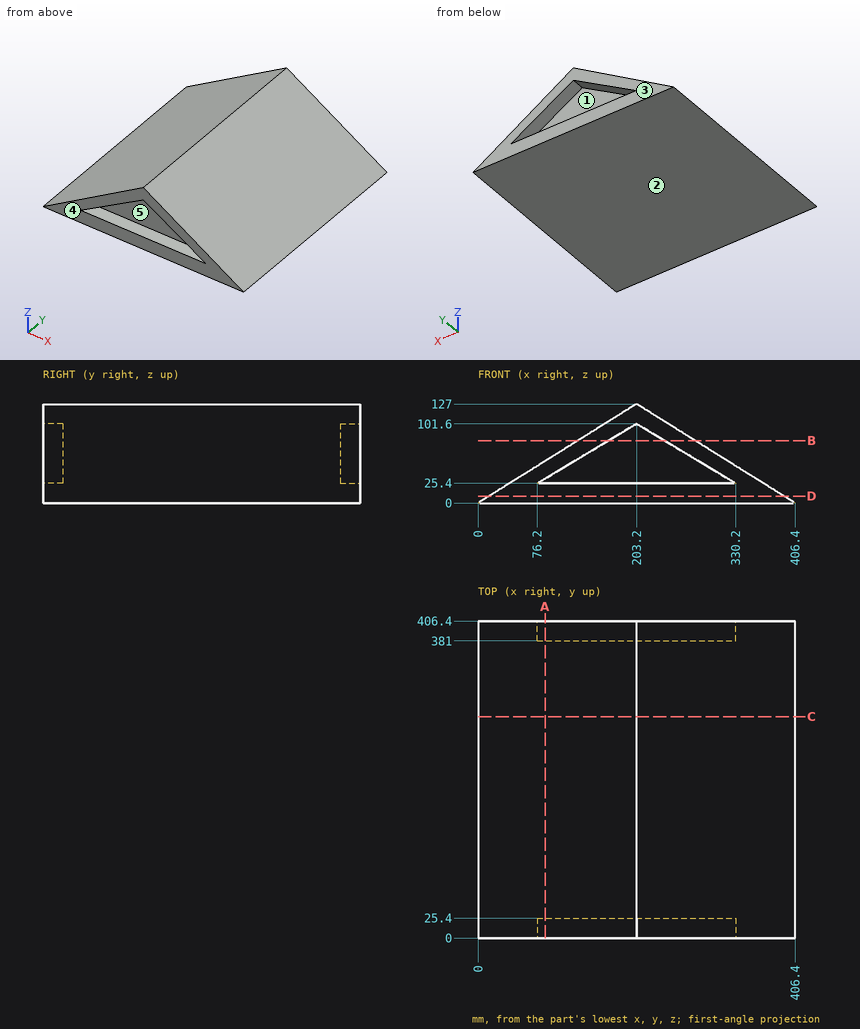
Geometry check sheet. Reference: drawing and pictorial views, mm from the part's lowest x, y, z. A direction names the side the tool comes from. Round coordinates to 2 decimals unless told otherwise and drop trailing zeros. Write each loop counter-clockwise with the first axis right and the second up, starting at its lowest first coordinate (ties: lowest second). Pieces come first, ordered by that corner, then holes.
(1) Material ranges on line 1 (Y direction, x = 214, z = 39.5); line 2 (X direction, y = 276, z = 67.5); line 3 (X direction, y = 189.5, z = 92.5), recorded low to high.
Returned:
line 1: y = 25.4 to 381
line 2: x = 108 to 298.4
line 3: x = 148 to 258.4
(2) Section check B-B (z = 80). Enter the section's corners in (x, y).
Returned:
outline: (128, 0) - (167.2, 0) - (167.2, 25.4) - (239.2, 25.4) - (239.2, 0) - (278.4, 0) - (278.4, 406.4) - (239.2, 406.4) - (239.2, 381) - (167.2, 381) - (167.2, 406.4) - (128, 406.4) - close
(3) Depth check by flat-ended pin: pin 1 Ø2 at (y, z) = (168, 34) entering from +X; pin 2 Ø10 at (x, z) = (219.5, 43) entering from -Y; pin 3 Ø8 at (x, y) = (273, 196.5) entering from +Z (3 decimals); pin 4 Ø10 at (x, z) = (144, 64) entering from -Y. Enter the tip coordinate at first touch or a pass-through.
Returned:
pin 1: stops at x = 353.6
pin 2: stops at y = 25.4
pin 3: stops at z = 85.875
pin 4: stops at y = 0
(4) Section check A-A (x = 86). Enter the section's corners in (y, z), plus the area to 3 significant figures.
Returned:
outline: (0, 0) - (406.4, 0) - (406.4, 25.4) - (381, 25.4) - (381, 31.28) - (406.4, 31.28) - (406.4, 53.75) - (0, 53.75) - (0, 31.28) - (25.4, 31.28) - (25.4, 25.4) - (0, 25.4) - close
area: 21,500 mm2
(5) Section check C-C (y = 284). Enter the section's corners in (x, z).
Returned:
outline: (0, 0) - (406.4, 0) - (203.2, 127) - close
(6) Mould release check, pull along Z, two halves, no side actions. Record for the marked faces 1, 2 and 3: pulls with the +Z half, pulls with the -Z half, needs draft (parallel to the pull), parting line crosses it, or undercut.
Returned:
face 1: undercut
face 2: pulls with the -Z half
face 3: needs draft
(7) Section check D-D (z = 9). Enter the section's corners in (x, y), plus the area to 3 significant figures.
Returned:
outline: (14.4, 0) - (392, 0) - (392, 406.4) - (14.4, 406.4) - close
area: 153,000 mm2
(8) Access from +Z, -Z, +X, -X, +Y, -Y to the whole of each face (thin tool, end or side, straight path). Record for the marked faces 4 and 5.
Returned:
face 4: +Z, -Z, +X, -X, -Y
face 5: -Y
